Work out the finished part from the listing and answer in its coordinate system (mm). A direction names the side the tool comes from. Coordinates: 2 decimals unless noted, no trailing zeros. Loops run counter-clockwise (first coordinate to the right, second up) from the corner with the lowest first, then second, coordinate; pieces in that order, holes last. Notation, with made-up numbers: (82, 60) -> (136, 60) arc R30 cw to (136, 82) -> close; hole circle Ø7 at (30, -3). An arc over 180 degrees is marked (long way). Answer as CSV lines item,"result".
```python
from build123d import *

# Parameters (mm, degrees)
SKETCH_1_W          = 41
SKETCH_1_H          = 69
EXTRUDE_1_DEPTH     = 1.6
SKETCH_3_R          = 2.5
CUT_EXTRUDE_1_DEPTH = 0.1
FILLET_4_R          = 3.5
SKETCH_4_R          = 1.5
CUT_EXTRUDE_2_DEPTH = 1.9
SKETCH_5_W          = 4.9
SKETCH_5_H          = 55
EXTRUDE_2_DEPTH     = 2.5
SKETCH_6_W          = 4.9
SKETCH_6_H          = 55
EXTRUDE_3_DEPTH     = 2.5
SKETCH_7_W          = 20
SKETCH_7_H          = 2.5
EXTRUDE_4_DEPTH     = 2.5
SKETCH_8_W          = 12.5
SKETCH_8_H          = 2.5
EXTRUDE_5_DEPTH     = 2.5
SKETCH_9_W          = 8
SKETCH_9_H          = 5
EXTRUDE_6_DEPTH     = 2.5
CUT_EXTRUDE_3_DEPTH = 4
EXTRUDE_7_DEPTH     = 1.5
SKETCH_12_W         = 3.5
SKETCH_12_H         = 53.5
EXTRUDE_8_DEPTH     = 6
SKETCH_13_W         = 3.5
SKETCH_13_H         = 53.5
EXTRUDE_9_DEPTH     = 6
SKETCH_14_W         = 18.5
SKETCH_14_H         = 1
EXTRUDE_10_DEPTH    = 6
SKETCH_15_W         = 11
SKETCH_15_H         = 1
EXTRUDE_11_DEPTH    = 6
SKETCH_16_W         = 3.5
SKETCH_16_H         = 53.5
SKETCH_16_W_2       = 18.5
SKETCH_16_H_2       = 1
SKETCH_16_W_3       = 11
EXTRUDE_12_DEPTH    = 1.5
SKETCH_17_R         = 2.5
CUT_EXTRUDE_4_DEPTH = 0.1
SKETCH_18_W         = 14
SKETCH_18_H         = 16
EXTRUDE_13_DEPTH    = 2.5
CUT_EXTRUDE_5_DEPTH = 15


with BuildPart() as part:
    # Эскиз1 → Бобышка-Вытянуть1 (new body)
    with BuildSketch(Plane(origin=(0, 0, 0), x_dir=(1, 0, 0), z_dir=(0, 1, 0))):
        with Locations((6.8125, -2.44375)):
            Rectangle(SKETCH_1_W, SKETCH_1_H)
    extrude(amount=EXTRUDE_1_DEPTH)

    # Эскиз3 → Вырез-Вытянуть1 (cut)
    with BuildSketch(Plane(origin=(0, 1.6, 0), x_dir=(1, 0, 0), z_dir=(0, 1, 0))):
        with Locations((-10.6875, 29.05625)):
            Circle(SKETCH_3_R)
        with Locations((24.3125, 29.05625)):
            Circle(SKETCH_3_R)
        with Locations((-10.6875, -33.94375)):
            Circle(SKETCH_3_R)
        with Locations((24.3125, -33.94375)):
            Circle(SKETCH_3_R)
    extrude(amount=-CUT_EXTRUDE_1_DEPTH, mode=Mode.SUBTRACT)

    # Скругление4
    fillet_4_edges = [part.edges().sort_by_distance(p)[0] for p in [
        (-13.6875, 0.8, -32.05625),
        (27.3125, 0.8, -32.05625),
        (27.3125, 0.8, 36.94375),
        (-13.6875, 0.8, 36.94375),
    ]]
    fillet(fillet_4_edges, radius=FILLET_4_R)

    # Эскиз4 → Вырез-Вытянуть2 (cut)
    with BuildSketch(Plane(origin=(0, 1.5, 0), x_dir=(1, 0, 0), z_dir=(0, 1, 0))):
        with Locations((-10.6875, 29.05625)):
            Circle(SKETCH_4_R)
        with Locations((24.3125, 29.05625)):
            Circle(SKETCH_4_R)
        with Locations((-10.6875, -33.94375)):
            Circle(SKETCH_4_R)
        with Locations((24.3125, -33.94375)):
            Circle(SKETCH_4_R)
    extrude(amount=-CUT_EXTRUDE_2_DEPTH, mode=Mode.SUBTRACT)

    # Эскиз5 → Бобышка-Вытянуть2 (add)
    with BuildSketch(Plane(origin=(0, 1.6, 0), x_dir=(1, 0, 0), z_dir=(0, 1, 0))):
        with Locations((-11.1375, -2.44375)):
            Rectangle(SKETCH_5_W, SKETCH_5_H)
    extrude(amount=EXTRUDE_2_DEPTH)

    # Эскиз6 → Бобышка-Вытянуть3 (add)
    with BuildSketch(Plane(origin=(0, 1.6, 0), x_dir=(1, 0, 0), z_dir=(0, 1, 0))):
        with Locations((24.7625, -2.44375)):
            Rectangle(SKETCH_6_W, SKETCH_6_H)
    extrude(amount=EXTRUDE_3_DEPTH)

    # Эскиз7 → Бобышка-Вытянуть4 (add)
    with BuildSketch(Plane(origin=(0, 1.6, 0), x_dir=(1, 0, 0), z_dir=(0, 1, 0))):
        with Locations((6.8125, 24.80625)):
            Rectangle(SKETCH_7_W, SKETCH_7_H)
    extrude(amount=EXTRUDE_4_DEPTH)

    # Эскиз8 → Бобышка-Вытянуть5 (add)
    with BuildSketch(Plane(origin=(0, 1.6, 0), x_dir=(1, 0, 0), z_dir=(0, 1, 0))):
        with Locations((13.0625, 29.80625)):
            Rectangle(SKETCH_8_W, SKETCH_8_H)
    extrude(amount=EXTRUDE_5_DEPTH)

    # Эскиз9 → Бобышка-Вытянуть6 (add)
    with BuildSketch(Plane(origin=(0, 1.6, 0), x_dir=(1, 0, 0), z_dir=(0, 1, 0))):
        with Locations((-1.6875, 30.30625)):
            Rectangle(SKETCH_9_W, SKETCH_9_H)
    extrude(amount=EXTRUDE_6_DEPTH)

    # Эскиз10 → Вырез-Вытянуть3 (cut)
    with BuildSketch(Plane(origin=(0, 0, -32.80625), x_dir=(-1, 0, 0), z_dir=(0, 0, -1))):
        with BuildLine():
            Line((-0.715104459, 3.393132584), (4.188395452, 3.393132584))
            ThreePointArc((4.188395452, 3.393132584), (4.827982397, 2.753545639), (4.188395452, 2.113958694))
            Line((4.188395452, 2.113958694), (-0.715104459, 2.113958694))
            ThreePointArc((-0.715104459, 2.113958694), (-1.354691404, 2.753545639), (-0.715104459, 3.393132584))
        make_face()
    extrude(amount=-CUT_EXTRUDE_3_DEPTH, mode=Mode.SUBTRACT)

    # Эскиз11 → Бобышка-Вытянуть7 (add)
    with BuildSketch(Plane(origin=(0, 1.6, 0), x_dir=(1, 0, 0), z_dir=(0, 1, 0))):
        Polygon((-2.1875, 0.05625), (6.651334765, 8.895084765), (15.49016953, 0.05625), (6.651334765, -8.782584765), align=None)
    extrude(amount=EXTRUDE_7_DEPTH)

    # Эскиз12 → Бобышка-Вытянуть8 (add)
    with BuildSketch(Plane(origin=(0, 4.1, 0), x_dir=(1, 0, 0), z_dir=(0, 1, 0))):
        with Locations((-11.1875, -2.44375)):
            Rectangle(SKETCH_12_W, SKETCH_12_H)
    extrude(amount=EXTRUDE_8_DEPTH)

    # Эскиз13 → Бобышка-Вытянуть9 (add)
    with BuildSketch(Plane(origin=(0, 4.1, 0), x_dir=(1, 0, 0), z_dir=(0, 1, 0))):
        with Locations((24.8125, -2.44375)):
            Rectangle(SKETCH_13_W, SKETCH_13_H)
    extrude(amount=EXTRUDE_9_DEPTH)

    # Эскиз14 → Бобышка-Вытянуть10 (add)
    with BuildSketch(Plane(origin=(0, 4.1, 0), x_dir=(1, 0, 0), z_dir=(0, 1, 0))):
        with Locations((6.8125, 24.80625)):
            Rectangle(SKETCH_14_W, SKETCH_14_H)
    extrude(amount=EXTRUDE_10_DEPTH)

    # Эскиз15 → Бобышка-Вытянуть11 (add)
    with BuildSketch(Plane(origin=(0, 4.1, 0), x_dir=(1, 0, 0), z_dir=(0, 1, 0))):
        with Locations((13.0625, 29.80625)):
            Rectangle(SKETCH_15_W, SKETCH_15_H)
    extrude(amount=EXTRUDE_11_DEPTH)

    # Эскиз16 → Бобышка-Вытянуть12 (add)
    with BuildSketch(Plane(origin=(0, 0, 0), x_dir=(-1, 0, 0), z_dir=(0, -1, 0))):
        with Locations((11.1875, -2.44375)):
            Rectangle(SKETCH_16_W, SKETCH_16_H)
        with Locations((-24.8125, -2.44375)):
            Rectangle(SKETCH_16_W, SKETCH_16_H)
        with Locations((-6.8125, 24.80625)):
            Rectangle(SKETCH_16_W_2, SKETCH_16_H_2)
        with Locations((-13.0625, 29.80625)):
            Rectangle(SKETCH_16_W_3, SKETCH_16_H_2)
    extrude(amount=EXTRUDE_12_DEPTH)

    # Эскиз17 → Вырез-Вытянуть4 (cut)
    with BuildSketch(Plane(origin=(0, 0, 0), x_dir=(-1, 0, 0), z_dir=(0, -1, 0))):
        with Locations((10.6875, -33.94375)):
            Circle(SKETCH_17_R)
        with Locations((-24.3125, -33.94375)):
            Circle(SKETCH_17_R)
        with Locations((10.6875, 29.05625)):
            Circle(SKETCH_17_R)
        with Locations((-24.3125, 29.05625)):
            Circle(SKETCH_17_R)
    extrude(amount=-CUT_EXTRUDE_4_DEPTH, mode=Mode.SUBTRACT)

    # Эскиз18 → Бобышка-Вытянуть13 (add)
    with BuildSketch(Plane(origin=(0, 1.6, 0), x_dir=(1, 0, 0), z_dir=(0, 1, 0))):
        with Locations((0.3125, -29.94375)):
            Rectangle(SKETCH_18_W, SKETCH_18_H)
    extrude(amount=EXTRUDE_13_DEPTH)

    # Эскиз19 → Вырез-Вытянуть5 (cut)
    with BuildSketch(Plane.XY.offset(37.94375)):
        with BuildLine():
            Line((-5.297012823, 3.809650009), (5.703882629, 3.809650009))
            ThreePointArc((5.703882629, 3.809650009), (6.599304352, 2.914228286), (5.703882629, 2.018806563))
            Line((5.703882629, 2.018806563), (-5.297012823, 2.018806563))
            ThreePointArc((-5.297012823, 2.018806563), (-6.192434546, 2.914228286), (-5.297012823, 3.809650009))
        make_face()
    extrude(amount=-CUT_EXTRUDE_5_DEPTH, mode=Mode.SUBTRACT)


solid = part.part
```
(1) For a pull along Z with two mould halves and no side action, classify faces 4 (the face through (22.312, 3, 3)), 5 (the face through (25, 3, 29.944)), 6 (the face through (7, 3, -26.056)) as pulls with the +Z half, pulls with the -Z half, needs draft (parallel to the pull), parting line crosses it, or undercut.
Computed values:
face 4,"needs draft"
face 5,"pulls with the +Z half"
face 6,"undercut"
(2) A cutting plane is placed at A-A, the plane y = 5.5. Write down the section's boundary in (x, z).
Computed values:
outline,"(-12.94, -24.31) -> (-9.44, -24.31) -> (-9.44, 29.19) -> (-12.94, 29.19) -> close; (-2.44, -25.31) -> (16.06, -25.31) -> (16.06, -24.31) -> (-2.44, -24.31) -> close; (7.56, -30.31) -> (18.56, -30.31) -> (18.56, -29.31) -> (7.56, -29.31) -> close; (23.06, -24.31) -> (26.56, -24.31) -> (26.56, 29.19) -> (23.06, 29.19) -> close"
(3) Which of the six approach directions +Z, -Z, +X, -X, +Y, -Y give full straight-line access (tool end or side, diameter ignored) to faces 1 (the face through (7, 3.1, 0)), 2 (the face through (7, 1, 36.944)), 3 (the face through (13, 7, -29.306))?
Computed values:
face 1,"+Y"
face 2,"+Z, +X, -X, -Y"
face 3,"+X, -X, +Y"
(4) A cutting plane is placed at B-B, the plane z = -13. Write down the section's boundary in (x, y).
Computed values:
outline,"(-13.69, 0) -> (-12.94, 0) -> (-12.94, -1.5) -> (-9.44, -1.5) -> (-9.44, 0) -> (23.06, 0) -> (23.06, -1.5) -> (26.56, -1.5) -> (26.56, 0) -> (27.31, 0) -> (27.31, 1.6) -> (27.21, 1.6) -> (27.21, 4.1) -> (26.56, 4.1) -> (26.56, 10.1) -> (23.06, 10.1) -> (23.06, 4.1) -> (22.31, 4.1) -> (22.31, 1.6) -> (-8.69, 1.6) -> (-8.69, 4.1) -> (-9.44, 4.1) -> (-9.44, 10.1) -> (-12.94, 10.1) -> (-12.94, 4.1) -> (-13.59, 4.1) -> (-13.59, 1.6) -> (-13.69, 1.6) -> close"
(5) Consider line 1 along X through (y, z) = (7.5, -21); line 2 along Y through (x, z) = (3, 26); line 3 along X through (y, z) = (3.75, 16). Determine where each line is inside the solid, lowest interval first.
Computed values:
line 1,"-12.94 to -9.44, 23.06 to 26.56"
line 2,"0 to 2.02, 3.81 to 4.1"
line 3,"-13.59 to -8.69, 22.31 to 27.21"
(6) Flat-ended cylindrical pins translate along their axes: pin 1 Ø4 at (x, z) = (23.5, -30.5) entering from -Y; pin 2 Ø0.8 at (y, z) = (7.5, -24.5) entering from -X; pin 3 Ø6 at (y, z) = (7, 1.5) entering from +X. Find the tip coordinate at first contact, or state that the pin passes through.
Computed values:
pin 1,"y = 0"
pin 2,"x = -12.94"
pin 3,"x = 27.21"
